Autodesk Inventor part; units mm, degrees
ref_plane "YZ Plane" through (0, 0, 0) normal (1, 0, 0) x (0, 1, 0)
ref_plane "XZ Plane" through (0, 0, 0) normal (0, 1, 0) x (-1, 0, 0)
ref_plane "XY Plane" through (0, 0, 0) normal (0, 0, 1) x (1, 0, 0)
sketch "Эскиз1" plane through (0, 0, 0) normal (0, 1, 0) x (-1, 0, 0)
  line L0 (0, 0) -> (97.5, 0)
  line L1 (97.5, 0) -> (97.5, -9)
  line L2 (97.5, -9) -> (75, -9)
  line L3 (75, -9) -> (75, -15)
  line L4 (0, -4) -> (0, 0)
  line L5 (75, -15) -> (69, -15)
  line L6 (69, -15) -> (69, -4)
  line L7 (69, -4) -> (0, -4)
  dimension "d0" = 195
  dimension "d1" = 150
  dimension "d3" = 9
  dimension "d5" = 15
  dimension "d6" = 138
  dimension "d7" = 4
revolve "Вращение1" add sketch "Эскиз1" angle 360 about axis through (0, 0, -4) along (0, 0, 1)
sketch "Эскиз3" plane through (0, 0, 0) normal (0, 0, 1) x (1, 0, 0)
  circle A0 centre (0, 0) radius 86.25 construction
  line L0 (0, 0) -> (-91.162, -91.162) construction
  line L1 (0, 0) -> (128.9225, 0) construction
  point P0 (0, 0)
  point P1 (-60.988, -60.988)
  point P2 (60.988, -60.988)
  point P3 (60.988, 60.988)
  point P4 (-60.988, 60.988)
  dimension "d15" = 172.5
  dimension "d16" = 135
  dimension "d19" = 360
hole "Отверстие1" at (-60.988, -60.988, 0) at (60.988, -60.988, 0) at (60.988, 60.988, 0) at (-60.988, 60.988, 0) direction (0, 0, -1) diameter 8.376 end through all
chamfer "Фаска1" distance 2 angle 45 2 edges at (75, 0, -15) (97.5, 0, 0)
sketch "Эскиз4" plane through (0, 0, 0) normal (0, 0, 1) x (1, 0, 0)
  circle A0 centre (0, 0) radius 97.5
  point P0 (0, 0)
hole "Отверстие2" at (0, 0, 0) direction (0, 0, -1) diameter 85 end through all
properties part number "МПСТ Крышка подшипника с отверстием 150" material "Сталь, углеродистая"
Geometry: final body of the model. Coordinates: model frame, mm. A direction names the side the tool comes from. Give positions to 0.01 mm unless a question says otherwise; leave off trailing zeros. Write each loop counter-clockwise with the first axis right and the second up, starting at its lowest first coordinate (ties: lowest second). Pieces come first, ordered by that corner, then holes.
(1) First-contact query: P1, Ø3, axis at y = -72.5, z = -3, coming from the +X side; P2, Ø7.5, axis at x = 60.988, y = 60.988, coming from the -Z side; P3, Ø1.5, axis at x = -51, y = -31.5, coming from the -Z side; P4, Ø1, axis at y = -36.5, z = -3.5, coming from the -X side. Flat tips, straight axial feed; report the tip coordinate or a pass-through.
(2) Cut plane A-A, the plane x = 0. Return loops of the section in (y, z).
(3) Ray query, line 1 (Y direction, x = 0, z = -5); line 2 (Y direction, x = -59, z = -1.25). Return the intervals inside material, ascending.
(4) Access query for faces 1 (the cylindrical face through (-63.82, -57.9, -4.56)), 2 (the flat face through (32, 30, -4)). Directions: +Z, -Z, +X, -X, +Y, -Y. A direction counts if a zero-diameter tool reaches every point of the face in a straight line with its end or side. Return the directions, or none.
(5) Mould query, pull axis X, two halves, no side actions, for faces 3 (the flat face through (44, -1, 0)), 4 (the cylindrical face through (-65.14, 61.53, -4.56)), 5 (the cylindrical face through (9.764, 74.362, -11.028)). Classes: released by +X, released by -X, zero draft, split by the parting line, or undercut.
Values follow:
1. P1: stops at x = 66.82
1. P2: passes through
1. P3: stops at z = -4
1. P4: stops at x = -90.61
2. outline: (-97.5, -9) - (-75, -9) - (-75, -13) - (-73, -15) - (-69, -15) - (-69, -4) - (-42.5, -4) - (-42.5, 0) - (-95.5, 0) - (-97.5, -2) - close; (42.5, -4) - (69, -4) - (69, -15) - (73, -15) - (75, -13) - (75, -9) - (97.5, -9) - (97.5, -2) - (95.5, 0) - (42.5, 0) - close
3. line 1: y = -97.5 to -69, 69 to 97.5
3. line 2: y = -76.68 to -64.67, -57.3 to 57.3, 64.67 to 76.68
4. face 1: +Z, -Z
4. face 2: -Z
5. face 3: zero draft
5. face 4: undercut
5. face 5: split by the parting line
